Autodesk Inventor part; units mm, degrees
ref_plane "YZ Plane" through (0, 0, 0) normal (1, 0, 0) x (0, 1, 0)
ref_plane "XZ Plane" through (0, 0, 0) normal (0, 1, 0) x (-1, 0, 0)
ref_plane "XY Plane" through (0, 0, 0) normal (0, 0, 1) x (1, 0, 0)
sketch "Sketch1" plane through (0, 0, 0) normal (0, 0, 1) x (1, 0, 0)
  line L0 (-4.5, 0) -> (-4.5, 15)
  line L1 (-4.5, 15) -> (-2.5, 15)
  line L2 (-2.5, 15) -> (-2.5, 14)
  line L3 (-2.5, 14) -> (2.5, 14)
  line L4 (2.5, 14) -> (2.5, 15)
  line L5 (2.5, 15) -> (4.5, 15)
  line L6 (4.5, 15) -> (4.5, 0)
  line L7 (4.5, 0) -> (-4.5, 0)
  line L8 (4.5, 8) -> (5.5, 8)
  line L9 (5.5, 8) -> (5.5, 0)
  line L10 (4.5, 0) -> (5.5, 0)
  line L11 (0, 14) -> (0, 0) construction
  dimension "d0" = 30
  dimension "d1" = 2
  dimension "d2" = 2
  dimension "d3" = 9
  dimension "d4" = 16
  dimension "d5" = 1
  dimension "d6" = 28
revolve "Revolution1" add sketch "Sketch1" angle 360 about axis through (4.5, 0, 0) along (-1, 0, 0)
sketch "Sketch3" plane through (-4.5, 0, 0) normal (-1, 0, 0) x (0, 0, 1)
  circle A0 centre (0, 0) radius 15
  point P0 (0, 0)
hole "Hole2" at (-4.5, 0, 0) direction (1, 0, 0) diameter 4.134 depth 10
sketch "Sketch4" plane through (5.5, 0, 0) normal (1, 0, 0) x (0, 0, -1)
  circle A0 centre (0, 0) radius 8
  point P0 (0, 0)
hole "Hole3" at (5.5, 0, 0) direction (-1, 0, 0) diameter 10 depth 9
fillet "Fillet2" radius 1 2 edges at (-4.5, -15, 0) (4.5, -15, 0)
properties part number "11 base"
Can you work these out from the model? Positions are in its coordinate system, mm. A direction names the side the tool comes from. Coordinates: 2 decimals unless noted, no trailing zeros. Order: outer loops, then holes, each group sorted by start corner. A loop starts at its lowest first (then second) coordinate and runs counter-clockwise, first axis right, second up. Notation, with made-up numbers: (12, -39) - (19, -39) arc R24 cw to (19, -14) - close; hole circle Ø10 at (-9.75, 82). An arc over 180 degrees is marked (long way). Answer in a Markdown table with one row per item.
1. If I drill on line 1 along Z through (x, y) = (-0.5, 0); line 2 along X through (y, z) = (-11.5, -5.25), over which ranges is the centre line in solid material (lowest first)?
Reply:
| item | result |
|---|---|
| line 1 | z = -14 to -5, 5 to 14 |
| line 2 | x = -4.5 to 4.5 |
2. Suppose I cut it at A-A (y = 0). Please give me the cut outline in (x, z).
Reply:
| item | result |
|---|---|
| outline | (-4.5, -14) arc R1 ccw to (-3.5, -15) - (-2.5, -15) - (-2.5, -14) - (2.5, -14) - (2.5, -15) - (3.5, -15) arc R1 ccw to (4.5, -14) - (4.5, -8) - (5.5, -8) - (5.5, -5) - (-3.5, -5) - (-3.5, -2.07) - (-4.5, -2.07) - close; (-4.5, 2.07) - (-3.5, 2.07) - (-3.5, 5) - (5.5, 5) - (5.5, 8) - (4.5, 8) - (4.5, 14) arc R1 ccw to (3.5, 15) - (2.5, 15) - (2.5, 14) - (-2.5, 14) - (-2.5, 15) - (-3.5, 15) arc R1 ccw to (-4.5, 14) - close |
3. Suppose I cut it at C-C (x = -1). Please give me the cut outline in (y, z), and give its area (3 significant figures).
Reply:
| item | result |
|---|---|
| outline | circle Ø28 at (0, 0); hole circle Ø10 at (0, 0) |
| area | 537 mm^2 |
4. If we mould it in two halves opening along Z, with no side actions, what happens to faces 4 (the cylindrical face through (-3.99, 1.26, -1.64)), 5 (the cylindrical face through (5.01, -1.73, -7.81)), 6 (the flat face through (5.5, -0.1, 5.2))? For each: pulls with the +Z half, pulls with the -Z half, needs draft (parallel to the pull), parting line crosses it, or undercut.
Reply:
| item | result |
|---|---|
| face 4 | undercut |
| face 5 | parting line crosses it |
| face 6 | needs draft |
5. For faces 1 (the flat face through (4.5, 6, 6)), 2 (the cylindrical face through (0.035, 12.932, -5.362)), 3 (the cylindrical face through (3.007, -14.985, 0.66)), which set-ups out of +Z, -Z, +X, -X, +Y, -Y let a thin tool reach every point of the face, with its end or its side?
Reply:
| item | result |
|---|---|
| face 1 | +X |
| face 2 | none |
| face 3 | +X, -X |
6. For pin 1 (1.5 mm diameter, centred on x = -0.5, y = -10.5, fed in from -Z); pin 2 (3 mm diameter, centred on y = -1, z = 2.5, fed in from +X); pin 3 (5 mm diameter, centred on x = -1, z = 5.5, fed in from -Y), each with a flat end and sliding along its axis, tell me the tip position at first contact or that it passes through.
Reply:
| item | result |
|---|---|
| pin 1 | stops at z = -10.05 |
| pin 2 | stops at x = -3.5 |
| pin 3 | stops at y = -14.59 |
